Work out the finished part from the listing and answer in its coordinate system (mm). A direction names the side the tool comes from. Round coordinates to 2 decimals unless told otherwise and drop trailing zeros. Order: outer loops, then holes, each group sorted by start corner. A loop starts at its lowest first (then second) coordinate and runs counter-clockwise, first axis right, second up. Notation, with made-up numbers: (76.5, 21.5) - (112.5, 21.5) arc R34 cw to (112.5, 52.5) - close; hole circle Ø11 at (78, 61.5). An arc over 180 degrees is marked (long way). Put each result on its own line as item: value.
```python
from build123d import *

# Parameters (mm, degrees)
CROQUIS1_W                    = 50.8
CROQUIS1_H                    = 25.4
CROQUIS1_W_2                  = 47.8
CROQUIS1_H_2                  = 22.4
SALIENTE_EXTRUIR1_DEPTH       = 450
CROQUIS2_R                    = 11.5
CROQUIS2_R_2                  = 2
CORTAR_EXTRUIR1_DEPTH         = 26
TALADRO_DE_MARGEN_PARA_1_41_D = 6.7564
CROQUIS5_R                    = 6
CROQUIS5_R_2                  = 2.5
CORTAR_EXTRUIR2_DEPTH         = 25.4


with BuildPart() as part:
    # Croquis1 → Saliente-Extruir1 (new body)
    with BuildSketch(Plane.XY):
        Rectangle(CROQUIS1_W, CROQUIS1_H)
        Rectangle(CROQUIS1_W_2, CROQUIS1_H_2, mode=Mode.SUBTRACT)
    extrude(amount=SALIENTE_EXTRUIR1_DEPTH)

    # Croquis2 → Cortar-Extruir1 (cut)
    with BuildSketch(Plane(origin=(0, -12.7, 0), x_dir=(-1, 0, 0), z_dir=(0, -1, 0))):
        with Locations((0, -387.5)):
            Circle(CROQUIS2_R)
        with Locations((15.5, -403)):
            Circle(CROQUIS2_R_2)
        with Locations((-15.5, -403)):
            Circle(CROQUIS2_R_2)
        with Locations((-15.5, -372)):
            Circle(CROQUIS2_R_2)
        with Locations((15.5, -372)):
            Circle(CROQUIS2_R_2)
    extrude(amount=-CORTAR_EXTRUIR1_DEPTH, mode=Mode.SUBTRACT)

    # Taladro de margen para 1/41 (through all)
    with Locations(Plane(origin=(-25.4, 197.888619806, 162.989101594), x_dir=(0, -1, 0), z_dir=(-1, 0, 0))):
        with Locations((197.488619806, 269.010898406), (197.488619806, 178.010898406), (197.488619806, 144.010898406), (572.888619806, 144.010898406), (572.888619806, 178.010898406), (572.888619806, 269.010898406)):
            Hole(TALADRO_DE_MARGEN_PARA_1_41_D / 2)

    # Croquis5 → Cortar-Extruir2 (cut)
    with BuildSketch(Plane.XZ.offset(12.7)):
        with Locations((14.9, 298.5)):
            Circle(CROQUIS5_R)
        with Locations((14.9, 316.2)):
            Circle(CROQUIS5_R_2)
        with Locations((14.9, 280.8)):
            Circle(CROQUIS5_R_2)
    extrude(amount=-CORTAR_EXTRUIR2_DEPTH, mode=Mode.SUBTRACT)


solid = part.part
```
1) A cutting plane is placed at B-B on z = 222. Write down the section's boundary in (x, y).
Findings below:
outline: (-25.4, -12.7) - (25.4, -12.7) - (25.4, 12.7) - (-25.4, 12.7) - close; hole (-23.9, -11.2) - (23.9, -11.2) - (23.9, 11.2) - (-23.9, 11.2) - close
2) Given pin 1 Ø2.5 at (x, z) = (-15.5, 372) entering from +Y, flat-ended and moving along its own axis, determine where the tip first touches the part or whether it passes through.
Findings below:
pin 1: passes through
3) A cutting plane is placed at A-A on z = 298.5. Write down the section's boundary in (x, y), then the cut area to 3 significant figures.
Findings below:
outline: (-25.4, -12.7) - (8.9, -12.7) - (8.9, -11.2) - (-23.9, -11.2) - (-23.9, 11.2) - (8.9, 11.2) - (8.9, 12.7) - (-25.4, 12.7) - close; (20.9, -12.7) - (25.4, -12.7) - (25.4, 12.7) - (20.9, 12.7) - (20.9, 11.2) - (23.9, 11.2) - (23.9, -11.2) - (20.9, -11.2) - close
area: 184 mm2
4) For faces 1 (the flat face through (0, 11.2, 222)), 2 (the flat face through (0, -12, 0)), determine the directions among +Z, -Z, +X, -X, +Y, -Y from which every point of the face is accessible in a straight line to the end or side of a thin tool.
Findings below:
face 1: +Z, -Z
face 2: -Z, +X, -X, +Y, -Y
5) Straight lines are drawn through the part: L1, parallel to Z at x = -24.45, y = 0.4; L2, parallel to X at y = 11.75, z = 372; L3, parallel to X at y = 9.25, z = 89. For each, find the intervals that lie inside material, in ascending order. Write a range as from..to.
Findings below:
L1: z = 0..303.62, 310.38..337.62, 344.38..428.62, 435.38..450
L2: x = -25.4..-17.5, -13.5..13.5, 17.5..25.4
L3: x = -25.4..-23.9, 23.9..25.4
6) A cutting plane is placed at D-D on z = 387.5. Write down the section's boundary in (x, y), then the cut area to 3 significant figures.
Findings below:
outline: (-25.4, -12.7) - (-11.5, -12.7) - (-11.5, -11.2) - (-23.9, -11.2) - (-23.9, 11.2) - (-11.5, 11.2) - (-11.5, 12.7) - (-25.4, 12.7) - close; (11.5, -12.7) - (25.4, -12.7) - (25.4, 12.7) - (11.5, 12.7) - (11.5, 11.2) - (23.9, 11.2) - (23.9, -11.2) - (11.5, -11.2) - close
area: 151 mm2
7) For a pull along Y with two mould halves and no side action, classify faces 3 (the flat face through (0, 12.7, 222)), 4 (the flat face through (-23.9, 0, 222)), 5 (the flat face through (-25.4, 0, 222)), 6 (the flat face through (0, -11.2, 222)) as pulls with the +Y half, pulls with the -Y half, needs draft (parallel to the pull), parting line crosses it, or undercut.
Findings below:
face 3: pulls with the +Y half
face 4: undercut
face 5: needs draft
face 6: undercut
8) A cutting plane is placed at C-C on x = -0.5. Write down the section's boundary in (y, z), then the cut area to 3 significant figures.
Findings below:
outline: (-12.7, 0) - (-11.2, 0) - (-11.2, 376.01) - (-12.7, 376.01) - close; (-12.7, 398.99) - (-11.2, 398.99) - (-11.2, 450) - (-12.7, 450) - close; (11.2, 0) - (12.7, 0) - (12.7, 376.01) - (11.2, 376.01) - close; (11.2, 398.99) - (12.7, 398.99) - (12.7, 450) - (11.2, 450) - close
area: 1,280 mm2
